from build123d import *

# Parameters (mm, degrees)
BOSS_EXTRUDE1_DEPTH     = 38.1
SHELL1_T                = -2.54
CUT_EXTRUDE1_REACH      = 782.53
SKETCH3_W               = 33.02
SKETCH3_H               = 33.02
BOSS_EXTRUDE2_DEPTH     = 2.54
SKETCH5_R               = 6.35
CUT_EXTRUDE2_DEPTH      = 575.603362093
SKETCH7_W               = 38.1
SKETCH7_H               = 38.1
SKETCH7_W_2             = 33.02
SKETCH7_H_2             = 33.02
BOSS_EXTRUDE3_DEPTH     = 127
CUT_EXTRUDE4_REACH      = 620.716
SKETCH8_R               = 6.35
CUT_EXTRUDE6_DEPTH      = 644.98208109
CUT_EXTRUDE6_DEPTH_BACK = 644.98208109
CUT_EXTRUDE7_REACH      = 646.127
SKETCH11_R              = 6.35


with BuildPart() as part:
    # Sketch1 → Boss-Extrude1 (new body)
    with BuildSketch(Plane.XY):
        with BuildLine():
            Line((102.652877862, 330.2), (227.30280098, 114.3))
            ThreePointArc((227.30280098, 114.3), (227.30280098, 38.1), (161.311665212, 0))
            Line((161.311665212, 0), (-468.706063252, 0))
            Line((-468.706063252, 0), (-468.706063252, 38.1))
            Line((-468.706063252, 38.1), (161.311665212, 38.1))
            ThreePointArc((161.311665212, 38.1), (194.307233096, 57.15), (194.307233096, 95.25))
            Line((194.307233096, 95.25), (69.657309978, 311.15))
            Line((69.657309978, 311.15), (102.652877862, 330.2))
        make_face()
    extrude(amount=-BOSS_EXTRUDE1_DEPTH)

    # Shell1
    shell1_openings = [part.faces().sort_by_distance(p)[0] for p in [
        (86.15509392, 320.675, -19.05),
    ]]
    offset(amount=SHELL1_T, openings=shell1_openings, kind=Kind.INTERSECTION)

    # Sketch3 → Cut-Extrude1 (cut, up to next)
    with BuildSketch(Plane.ZY.offset(468.706063252), mode=Mode.PRIVATE) as cut_extrude1_sk1:
        with Locations((-19.05, 19.05)):
            Rectangle(SKETCH3_W, SKETCH3_H)
    cut_extrude1_tool1 = extrude(cut_extrude1_sk1.sketch, amount=-CUT_EXTRUDE1_REACH, mode=Mode.PRIVATE) & part.part
    add(cut_extrude1_tool1.solids().sort_by_distance((-468.706063, 19.05, -19.05))[0], mode=Mode.SUBTRACT)

    # Sketch4 → Boss-Extrude2 (add)
    with BuildSketch(Plane.XY):
        Polygon((2.178975516, 38.1), (144.901761863, 180.822786347), (196.194281247, 91.981536726), (142.31274452, 38.1), align=None)
    extrude(amount=-BOSS_EXTRUDE2_DEPTH)

    # Sketch5 → Cut-Extrude2 (cut, through all)
    with BuildSketch(Plane.XY):
        with Locations((-62.306063252, 19.05)):
            Circle(SKETCH5_R)
        with Locations((-290.906063252, 19.05)):
            Circle(SKETCH5_R)
        with Locations((-341.706063252, 19.05)):
            Circle(SKETCH5_R)
    extrude(amount=-CUT_EXTRUDE2_DEPTH, mode=Mode.SUBTRACT)

    # Sketch7 → Boss-Extrude3 (add)
    with BuildSketch(Plane(origin=(-117.317574699, 203.2, 0), x_dir=(0.8660254037844362, 0.5000000000000044, 0), z_dir=(-0.5000000000000044, 0.8660254037844362, 0))):
        with Locations((234.95, 19.05)):
            Rectangle(SKETCH7_W, SKETCH7_H)
        with Locations((234.95, 19.05)):
            Rectangle(SKETCH7_W_2, SKETCH7_H_2, mode=Mode.SUBTRACT)
    extrude(amount=BOSS_EXTRUDE3_DEPTH)

    # Sketch8 → Cut-Extrude4 (cut, up to next)
    with BuildSketch(Plane(origin=(0, 38.1, 0), x_dir=(1, 0, 0), z_dir=(0, 1, 0)), mode=Mode.PRIVATE) as cut_extrude4_sk1:
        with Locations(Location((-443.306063252, 19.05, 0), (0, 0, 180))):
            Circle(SKETCH8_R)
    cut_extrude4_tool1 = extrude(cut_extrude4_sk1.sketch, amount=-CUT_EXTRUDE4_REACH, mode=Mode.PRIVATE) & part.part
    add(cut_extrude4_tool1.solids().sort_by_distance((-443.306063, 38.1, -19.05))[0], mode=Mode.SUBTRACT)

    # Sketch10 → Cut-Extrude6 (cut, two sides: drawn at the far end of the back side and taken through both)
    with BuildSketch(Plane(origin=(0, 0, -2.54), x_dir=(-1, 0, 0), z_dir=(0, 0, -1)).offset(-CUT_EXTRUDE6_DEPTH_BACK)):
        with BuildLine():
            Line((-68.291720036, 57.15), (-119.091720036, 57.15))
            ThreePointArc((-119.091720036, 57.15), (-125.441720036, 50.8), (-119.091720036, 44.45))
            Line((-119.091720036, 44.45), (-68.291720036, 44.45))
            ThreePointArc((-68.291720036, 44.45), (-61.941720036, 50.8), (-68.291720036, 57.15))
        make_face()
        with BuildLine():
            Line((-68.291720036, 72.39), (-119.091720036, 72.39))
            ThreePointArc((-119.091720036, 72.39), (-125.441720036, 66.04), (-119.091720036, 59.69))
            Line((-119.091720036, 59.69), (-68.291720036, 59.69))
            ThreePointArc((-68.291720036, 59.69), (-61.941720036, 66.04), (-68.291720036, 72.39))
        make_face()
        with BuildLine():
            Line((-68.291720036, 87.63), (-119.091720036, 87.63))
            ThreePointArc((-119.091720036, 87.63), (-125.441720036, 81.28), (-119.091720036, 74.93))
            Line((-119.091720036, 74.93), (-68.291720036, 74.93))
            ThreePointArc((-68.291720036, 74.93), (-61.941720036, 81.28), (-68.291720036, 87.63))
        make_face()
    extrude(amount=CUT_EXTRUDE6_DEPTH + CUT_EXTRUDE6_DEPTH_BACK, mode=Mode.SUBTRACT)

    # Sketch11 → Cut-Extrude7 (cut, up to next)
    with BuildSketch(Plane.XY, mode=Mode.PRIVATE) as cut_extrude7_sk1:
        with Locations((35.366501125, 408.643423165)):
            Circle(SKETCH11_R)
    cut_extrude7_tool1 = extrude(cut_extrude7_sk1.sketch, amount=-CUT_EXTRUDE7_REACH, mode=Mode.PRIVATE) & part.part
    add(cut_extrude7_tool1.solids().sort_by_distance((35.366501, 408.643423, 0))[0], mode=Mode.SUBTRACT)


solid = part.part
The model under review builds one solid part; all positions refer to its coordinate system, in mm. A direction names the side the tool comes from. Give positions to 0.01 mm unless a question says otherwise; leave off trailing zeros. Write each loop counter-clockwise with the first axis right and the second up, starting at its lowest first coordinate (ties: lowest second). Pieces come first, ordered by that corner, then holes.
1. Add section A-A, the plane z = -19.05. Write out the cut boundary in (x, y), plus the area to 3 significant figures.
2. Tool access review of faces 4 (the flat face through (169.56, 65.35, -1.25)), 5 (the flat face through (-149, 2.54, -19)), 6 (the flat face through (132.345, 273.691, -18.819)): name each direction out of +Z, -Z, +X, -X, +Y, -Y from which nothing blocks a thin tool from reaching the whole face with its end or side.
3. Draft analysis for pull direction Z (two halves, no side actions). For faces 1 (the flat face through (134.545, 274.961, -18.783)), 2 (the flat face through (-50, 29, -38.1)), 3 (the flat face through (-52, 31, -35.56)), state which applies: +Z half, -Z half, draft (parallel to the pull), parting line (faces both ways), or undercut.
4. Wall thickness on L1, parallel to Y at x = -9, z = -6; L2, parallel to Y at x = 96, z = -30.5; L3, parallel to Y at x = 185, z = -34: over which ranges is each line inside the solid? List them lowest first.
5. For P1, Ø10, axis at x = -187, z = -26, coming from the +Y side; P2, Ø2, axis at x = 96, z = -1, coming from the -Y side; P3, Ø11.5, axis at x = -290.91, y = 19.05, coming from the -Z side; P4, Ø12, axis at y = 85, z = -34, coming from the -X side, all flat-tipped, find the tip position at first contact; note any pin that passes through.
6. Add section B-B, the plane x = -356.5. Write out the cut boundary in (y, z), plus the area to 3 significant figures.
7. Add section C-C, the plane y = 212. Write out the cut boundary in (x, z), plus the area to 3 significant figures.
Worked answers:
1. outline: (-468.71, 0) - (161.31, 0) arc R76.2 ccw to (227.3, 114.3) - (39.15, 440.19) - (36.95, 438.92) - (225.1, 113.03) arc R73.66 cw to (161.31, 2.54) - (-468.71, 2.54) - close; (-468.71, 35.56) - (-449.66, 35.56) - (-449.66, 38.1) - (-468.71, 38.1) - close; (-436.96, 35.56) - (161.31, 35.56) arc R40.64 ccw to (196.51, 96.52) - (8.36, 422.41) - (6.16, 421.14) - (194.31, 95.25) arc R38.1 cw to (161.31, 38.1) - (-436.96, 38.1) - close
1. area: 5,690 mm2
2. face 4: +Z, -Z
2. face 5: -X
2. face 6: none
3. face 1: draft
3. face 2: -Z half
3. face 3: undercut
4. L1: y = 0 to 2.54, 35.56 to 38.1
4. L2: y = 0 to 2.54, 35.56 to 38.1, 265.52 to 270.6, 336.64 to 341.72
4. L3: y = 3.78 to 6.45, 43.18 to 46.36, 111.37 to 116.45, 182.49 to 187.57
5. P1: stops at y = 38.1
5. P2: stops at y = 0
5. P3: passes through
5. P4: stops at x = 196.42
6. outline: (0, -38.1) - (38.1, -38.1) - (38.1, 0) - (0, 0) - close; hole (2.54, -35.56) - (35.56, -35.56) - (35.56, -2.54) - (2.54, -2.54) - close
6. area: 361 mm2
7. outline: (126.9, -38.1) - (170.9, -38.1) - (170.9, 0) - (126.9, 0) - close; hole (129.83, -35.56) - (167.96, -35.56) - (167.96, -2.54) - (129.83, -2.54) - close
7. area: 417 mm2
